from build123d import *

# Parameters (mm, degrees)
SKETCH_W        = 180
SKETCH_H        = 133.35
PAD_DEPTH       = 5
SKETCH001_W     = 20.2
SKETCH001_H     = 101.85
SKETCH001_W_2   = 30
SKETCH001_H_2   = 77
POCKET_DEPTH    = 1
SKETCH002_W     = 28
SKETCH002_H     = 75
POCKET001_DEPTH = 4
SKETCH003_R     = 5
POCKET002_DEPTH = 4
SKETCH004_R     = 5
POCKET003_DEPTH = 4
PAD001_DEPTH    = 75


with BuildPart() as part:
    # Sketch (on XY_Plane of Origin) → Pad (new body)
    with BuildSketch(Plane.XY):
        with Locations((-90, 66.675)):
            Rectangle(SKETCH_W, SKETCH_H)
        with BuildLine():
            ThreePointArc((-9.5, 130), (-12.5, 127), (-9.5, 124))
            Line((-9.5, 124), (-4.5, 124))
            ThreePointArc((-4.5, 124), (-1.5, 127), (-4.5, 130))
            Line((-9.5, 130), (-4.5, 130))
        make_face(mode=Mode.SUBTRACT)
        with BuildLine():
            ThreePointArc((-9.5, 98.25), (-12.5, 95.25), (-9.5, 92.25))
            Line((-9.5, 92.25), (-4.5, 92.25))
            ThreePointArc((-4.5, 92.25), (-1.5, 95.25), (-4.5, 98.25))
            Line((-9.5, 98.25), (-4.5, 98.25))
        make_face(mode=Mode.SUBTRACT)
        with BuildLine():
            ThreePointArc((-9.5, 85.55), (-12.5, 82.55), (-9.5, 79.55))
            Line((-9.5, 79.55), (-4.5, 79.55))
            ThreePointArc((-4.5, 79.55), (-1.5, 82.55), (-4.5, 85.55))
            Line((-9.5, 85.55), (-4.5, 85.55))
        make_face(mode=Mode.SUBTRACT)
        with BuildLine():
            ThreePointArc((-9.5, 53.8), (-12.5, 50.8), (-9.5, 47.8))
            Line((-9.5, 47.8), (-4.5, 47.8))
            ThreePointArc((-4.5, 47.8), (-1.5, 50.8), (-4.5, 53.8))
            Line((-9.5, 53.8), (-4.5, 53.8))
        make_face(mode=Mode.SUBTRACT)
        with BuildLine():
            ThreePointArc((-9.5, 41.1), (-12.5, 38.1), (-9.5, 35.1))
            Line((-9.5, 35.1), (-4.5, 35.1))
            ThreePointArc((-4.5, 35.1), (-1.5, 38.1), (-4.5, 41.1))
            Line((-9.5, 41.1), (-4.5, 41.1))
        make_face(mode=Mode.SUBTRACT)
        with BuildLine():
            ThreePointArc((-9.5, 9.35), (-12.5, 6.35), (-9.5, 3.35))
            Line((-9.5, 3.35), (-4.5, 3.35))
            ThreePointArc((-4.5, 3.35), (-1.5, 6.35), (-4.5, 9.35))
            Line((-9.5, 9.35), (-4.5, 9.35))
        make_face(mode=Mode.SUBTRACT)
    extrude(amount=PAD_DEPTH)

    # Sketch001 (on Face30 of Pad) → Pocket (cut)
    with BuildSketch(Plane.XY.offset(5)):
        with Locations((-50.1, 66.675)):
            Rectangle(SKETCH001_W, SKETCH001_H)
        with Locations((-90.1, 66.675)):
            Rectangle(SKETCH001_W, SKETCH001_H)
        with Locations((-135, 66.675)):
            Rectangle(SKETCH001_W_2, SKETCH001_H_2)
    extrude(amount=-POCKET_DEPTH, mode=Mode.SUBTRACT)

    # Sketch002 (on Face43 of Pocket) → Pocket001 (cut)
    with BuildSketch(Plane.XY.offset(4)):
        with Locations((-135, 66.675)):
            Rectangle(SKETCH002_W, SKETCH002_H)
    extrude(amount=-POCKET001_DEPTH, mode=Mode.SUBTRACT)

    # Sketch003 (on Face48 of Pocket001) → Pocket002 (cut)
    with BuildSketch(Plane.XY.offset(4)):
        with Locations((-90.1, 66.675)):
            Circle(SKETCH003_R)
        with Locations((-90.1, 81.675)):
            Circle(SKETCH003_R)
        with Locations((-90.1, 96.675)):
            Circle(SKETCH003_R)
        with Locations((-90.1, 111.675)):
            Circle(SKETCH003_R)
        with Locations((-90.1, 51.675)):
            Circle(SKETCH003_R)
        with Locations((-90.1, 36.675)):
            Circle(SKETCH003_R)
        with Locations((-90.1, 21.675)):
            Circle(SKETCH003_R)
    extrude(amount=-POCKET002_DEPTH, mode=Mode.SUBTRACT)

    # Sketch004 (on Face56 of Pocket002) → Pocket003 (cut)
    with BuildSketch(Plane.XY.offset(4)):
        with Locations((-50.1, 66.675)):
            Circle(SKETCH004_R)
        with Locations((-50.1, 81.675)):
            Circle(SKETCH004_R)
        with Locations((-50.1, 96.675)):
            Circle(SKETCH004_R)
        with Locations((-50.1, 111.675)):
            Circle(SKETCH004_R)
        with Locations((-50.1, 51.675)):
            Circle(SKETCH004_R)
        with Locations((-50.1, 36.675)):
            Circle(SKETCH004_R)
        with Locations((-50.1, 21.675)):
            Circle(SKETCH004_R)
    extrude(amount=-POCKET003_DEPTH, mode=Mode.SUBTRACT)

    # Sketch005 (on Face5 of Pocket003) → Pad001 (join)
    with BuildSketch(Plane.XY.offset(5)):
        Polygon((-32.4, 129.675), (-120, 129.675), (-120, 122.175), (-117.5, 122.175), (-117.5, 127.175), (-114.9, 127.175), (-114.9, 107.175), (-112.4, 107.175), (-112.4, 127.175), (-80, 127.175), (-80, 122.175), (-77.5, 122.175), (-77.5, 127.175), (-74.9, 127.175), (-74.9, 107.175), (-72.4, 107.175), (-72.4, 127.175), (-40, 127.175), (-40, 122.175), (-37.5, 122.175), (-37.5, 127.175), (-34.9, 127.175), (-34.9, 107.175), (-32.4, 107.175), align=None)
        Polygon((-32.4, 3.675), (-32.4, 26.175), (-34.9, 26.175), (-34.9, 6.175), (-37.5, 6.175), (-37.5, 11.175), (-40, 11.175), (-40, 6.175), (-72.4, 6.175), (-72.4, 26.175), (-74.9, 26.175), (-74.9, 6.175), (-77.5, 6.175), (-77.5, 11.175), (-80, 11.175), (-80, 6.175), (-112.4, 6.175), (-112.4, 26.175), (-114.9, 26.175), (-114.9, 6.175), (-117.5, 6.175), (-117.5, 11.175), (-120, 11.175), (-120, 3.675), align=None)
    extrude(amount=PAD001_DEPTH)


solid = part.part
Could you check a few things on this model? Use its own coordinates, in mm. A direction names the side the tool comes from. Coordinates: 2 decimals unless noted, no trailing zeros. Order: outer loops, then holes, each group sorted by start corner. A loop starts at its lowest first (then second) coordinate and runs counter-clockwise, first axis right, second up. Notation, with made-up numbers: (41.5, -17.5) -> (69.5, -17.5) arc R23 ccw to (69.5, 21.5) -> close; hole circle Ø11 at (64, 43.5). An arc over 180 degrees is marked (long way). One line per item, written item: value. Start each with the question number.
1) I'm going to push flat-ended pins straight in: pin 1 (10 mm diameter, centred on x = -100.5, z = 40.5, fed in from -Y) (3 decimals); pin 2 (12 mm diameter, centred on x = -19, y = 49.5, fed in from -Z); pin 3 (2.5 mm diameter, centred on y = 124, z = 54.5, fed in from +X); pin 4 (9 mm diameter, centred on x = -50.1, y = 36.675, fed in from +Z). Where does each tip first touch, or does it pass through?
2) Which directions (+Z, -Z, +X, -X, +Y, -Y) give clear straight access to the entire face, cutting with the end or side of a thin tool? Please do faces 1 (the flat face through (-97, 67, 4)), 2 (the cylindrical face through (-12.5, 6.4, 2.5)).
3) Imagine slicing it at D-D on x = -17. List the corners of the cut face in (y, z) for me, plus the area to 3 significant figures.
4) Imagine slicing it at A-A on y = 89. List the corners of the cut face in (x, z) for me, plus the area to 3 significant figures.
5) Imagine slicing it at B-B on x = -133. List the corners of the cut face in (y, z) for me (3 decimals).
6) If I drill on L1, parallel to X at y = 120, z = 50; L2, parallel to Y at x = -97, z = 9 (3 decimals); L3, parallel to Y at x = -78.5, z = 32.5 (3 decimals), over which ranges is the centre line in solid material (lowest first)? Write a range as [from, to].
7) Imagine slicing it at C-C on x = -50.1. Count the separate pieces of the cut face and the enclosed holes in it, plus the area to 3 significant figures.
Answer list:
1. pin 1: stops at y = 3.675
1. pin 2: stops at z = 0
1. pin 3: stops at x = -32.4
1. pin 4: passes through
2. face 1: +Z
2. face 2: +Z, -Z
3. outline: (0, 0) -> (133.35, 0) -> (133.35, 5) -> (0, 5) -> close
3. area: 667 mm2
4. outline: (-180, 0) -> (-149, 0) -> (-149, 4) -> (-150, 4) -> (-150, 5) -> (-180, 5) -> close; (-121, 0) -> (0, 0) -> (0, 5) -> (-40, 5) -> (-40, 4) -> (-60.2, 4) -> (-60.2, 5) -> (-80, 5) -> (-80, 4) -> (-100.2, 4) -> (-100.2, 5) -> (-120, 5) -> (-120, 4) -> (-121, 4) -> close
4. area: 718 mm2
5. outline: (0, 0) -> (29.175, 0) -> (29.175, 4) -> (28.175, 4) -> (28.175, 5) -> (0, 5) -> close; (104.175, 0) -> (133.35, 0) -> (133.35, 5) -> (105.175, 5) -> (105.175, 4) -> (104.175, 4) -> close
6. L1: x = [-114.9, -112.4], [-74.9, -72.4], [-34.9, -32.4]
6. L2: y = [3.675, 6.175], [127.175, 129.675]
6. L3: y = [3.675, 11.175], [122.175, 129.675]
7. separate pieces: 8
7. enclosed holes: 0
7. area: 660 mm2
